```python
from build123d import *

# Parameters (mm, degrees)
SKETCH1_W           = 46
SKETCH1_H           = 35.12
BOSS_EXTRUDE1_DEPTH = 13.2
SKETCH2_W           = 13.25
SKETCH2_H           = 5.33
CUT_EXTRUDE1_DEPTH  = 1.5
SKETCH5_W           = 13.25
SKETCH5_H           = 5.33
CUT_EXTRUDE2_DEPTH  = 1.5
SKETCH6_W           = 14
SKETCH6_H           = 3.726009738
CUT_EXTRUDE3_DEPTH  = 1.5
FILLET1_R           = 2


with BuildPart() as part:
    # Sketch1 → Boss-Extrude1 (new body)
    with BuildSketch(Plane(origin=(0, 0, 0), x_dir=(1, 0, 0), z_dir=(0, 1, 0))):
        Rectangle(SKETCH1_W, SKETCH1_H)
    extrude(amount=BOSS_EXTRUDE1_DEPTH)

    # Sketch2 → Cut-Extrude1 (cut)
    with BuildSketch(Plane(origin=(0, 0, -17.56), x_dir=(-1, 0, 0), z_dir=(0, 0, -1))):
        with Locations((-10.945153605, 8.923987955)):
            Rectangle(SKETCH2_W, SKETCH2_H)
    extrude(amount=-CUT_EXTRUDE1_DEPTH, mode=Mode.SUBTRACT)

    # Sketch5 → Cut-Extrude2 (cut)
    with BuildSketch(Plane(origin=(0, 0, -17.56), x_dir=(-1, 0, 0), z_dir=(0, 0, -1))):
        with Locations((10.446134444, 8.878725803)):
            Rectangle(SKETCH5_W, SKETCH5_H)
    extrude(amount=-CUT_EXTRUDE2_DEPTH, mode=Mode.SUBTRACT)

    # Sketch6 → Cut-Extrude3 (cut)
    with BuildSketch(Plane.XY.offset(17.56)):
        with Locations((0, 9.85493568)):
            Rectangle(SKETCH6_W, SKETCH6_H)
    extrude(amount=-CUT_EXTRUDE3_DEPTH, mode=Mode.SUBTRACT)

    # Fillet1
    fillet1_edges = [part.edges().sort_by_distance(p)[0] for p in [
        (-23, 6.6, -17.56),
        (23, 6.6, -17.56),
        (23, 6.6, 17.56),
        (-23, 6.6, 17.56),
    ]]
    fillet(fillet1_edges, radius=FILLET1_R)


solid = part.part
```
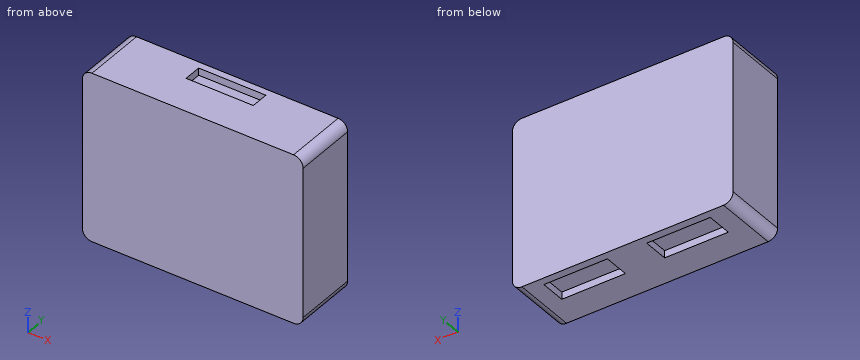
Part model, mm, in its own coordinate system. Coordinates: 2 decimals unless noted, no trailing zeros. Write each loop counter-clockwise with the first axis right and the second up, starting at its lowest first coordinate (ties: lowest second). Pieces come first, ordered by that corner, then holes.
Item 1: Slice it at C-C (y = 11). Write the cut outline in (x, z).
Item 2: Probe line 1 (Z direction, x = 12, y = 7.5); line 2 (X direction, y = 5, z = -16). List the from-to ranges inside material, lowest first.
Item 3: Pin check, flat tips, straight feed: pin 1 (1.6 mm diameter, centred on x = 14, z = -16.5, fed in from -Y); pin 2 (3 mm diameter, centred on x = -0.5, y = 10, fed in from +Z); pin 3 (0.8 mm diameter, centred on y = 9, z = -17, fed in from -X); pin 4 (1.2 mm diameter, centred on y = 10, z = -17, fed in from -X). Stop position of each tip, or through.
Item 4: Slice it at A-A (x = 9). Write the cut outline in (y, z).
Item 5: Slice it at B-B (y = 6.75). Write the cut outline in (x, z).
Results found:
1. outline: (-23, -15.56) arc R2 ccw to (-21, -17.56) - (-17.07, -17.56) - (-17.07, -16.06) - (-3.82, -16.06) - (-3.82, -17.56) - (4.32, -17.56) - (4.32, -16.06) - (17.57, -16.06) - (17.57, -17.56) - (21, -17.56) arc R2 ccw to (23, -15.56) - (23, 15.56) arc R2 ccw to (21, 17.56) - (7, 17.56) - (7, 16.06) - (-7, 16.06) - (-7, 17.56) - (-21, 17.56) arc R2 ccw to (-23, 15.56) - close
2. line 1: z = -16.06 to 17.56
2. line 2: x = -22.95 to 22.95
3. pin 1: stops at y = 0
3. pin 2: stops at z = 16.06
3. pin 3: stops at x = -22.71
3. pin 4: stops at x = -22.82
4. outline: (0, -17.56) - (6.26, -17.56) - (6.26, -16.06) - (11.59, -16.06) - (11.59, -17.56) - (13.2, -17.56) - (13.2, 17.56) - (0, 17.56) - close
5. outline: (-23, -15.56) arc R2 ccw to (-21, -17.56) - (-17.07, -17.56) - (-17.07, -16.06) - (-3.82, -16.06) - (-3.82, -17.56) - (4.32, -17.56) - (4.32, -16.06) - (17.57, -16.06) - (17.57, -17.56) - (21, -17.56) arc R2 ccw to (23, -15.56) - (23, 15.56) arc R2 ccw to (21, 17.56) - (-21, 17.56) arc R2 ccw to (-23, 15.56) - close
